Work out the finished part from the listing and answer in its coordinate system (mm). A direction names the side the tool comes from. Coordinates: 2 decimals unless noted, no trailing zeros. Loops run counter-clockwise (first coordinate to the right, second up) from the corner with the lowest first, then second, coordinate; pieces in that order, holes last. Notation, with made-up numbers: (-35.75, -19.5) -> (-30.75, -19.5) arc R33 cw to (-30.75, 16.5) -> close; hole circle Ø6 at (86, 25.25). An arc over 180 degrees is marked (long way). Use a Markdown table: item, result.
from build123d import *

# Parameters (mm, degrees)
SKETCH_R   = 11
SKETCH_R_2 = 2.5
PAD_DEPTH  = 1.3


with BuildPart() as part:
    # Sketch → Pad (new body)
    with BuildSketch(Plane.XY):
        with BuildLine():
            ThreePointArc((37.406136, 46.912482), (0, 60), (-37.406136, 46.912482))
            Line((-37.406136, 46.912482), (-31.633101, 40.032448))
            ThreePointArc((-33.931235, 38.104085), (-29.889624, 35.621067), (-31.633101, 40.032448))
            Line((-33.931235, 38.104085), (-39.704269, 44.98412))
            ThreePointArc((-39.704269, 44.98412), (0, -60), (39.704269, 44.98412))
            Line((33.931235, 38.104085), (39.704269, 44.98412))
            ThreePointArc((31.633101, 40.032448), (29.889624, 35.621067), (33.931235, 38.104085))
            Line((31.633101, 40.032448), (37.406136, 46.912482))
        make_face()
        Circle(SKETCH_R, mode=Mode.SUBTRACT)
        with Locations((0, 49)):
            Circle(SKETCH_R_2, mode=Mode.SUBTRACT)
        with Locations((48.25558, 8.508761)):
            Circle(SKETCH_R_2, mode=Mode.SUBTRACT)
        with Locations((42.435245, -24.5)):
            Circle(SKETCH_R_2, mode=Mode.SUBTRACT)
        with Locations((16.758987, -46.044938)):
            Circle(SKETCH_R_2, mode=Mode.SUBTRACT)
        with Locations((-16.758987, -46.044938)):
            Circle(SKETCH_R_2, mode=Mode.SUBTRACT)
        with Locations((-42.435245, -24.5)):
            Circle(SKETCH_R_2, mode=Mode.SUBTRACT)
        with Locations((-48.25558, 8.508761)):
            Circle(SKETCH_R_2, mode=Mode.SUBTRACT)
    extrude(amount=PAD_DEPTH)


solid = part.part
Q1. Section D-D on z = 0.35 is taken. State how many separate pieces and enclosed holes the cut face has, and give its area (3 significant figures).
Solved:
| item | result |
|---|---|
| separate pieces | 1 |
| enclosed holes | 8 |
| area | 10,700 mm² |
Q2. Section C-C on y = 43 is taken. Determine the outline of the cut face in (x, z), and give its area (3 significant figures).
Solved:
| item | result |
|---|---|
| outline | (-41.84, 0) -> (-38.04, 0) -> (-38.04, 1.3) -> (-41.84, 1.3) -> close; (-34.12, 0) -> (34.12, 0) -> (34.12, 1.3) -> (-34.12, 1.3) -> close; (38.04, 0) -> (41.84, 0) -> (41.84, 1.3) -> (38.04, 1.3) -> close |
| area | 98.6 mm² |
Q3. Determine the mould class of faces 1 (the cylindrical face through (-14.45, -47, 0.64)), 2 (the flat face through (12, 1, 0)), 3 (the cylindrical face through (0.565, 59.997, 0.641)) for opening direction Y: pulls with the +Y half, pulls with the -Y half, needs draft (parallel to the pull), parting line crosses it, or undercut.
Solved:
| item | result |
|---|---|
| face 1 | undercut |
| face 2 | needs draft |
| face 3 | pulls with the +Y half |
Q4. Section A-A on y = 0 is taken. Determine the outline of the cut face in (x, z).
Solved:
| item | result |
|---|---|
| outline | (-60, 0) -> (-11, 0) -> (-11, 1.3) -> (-60, 1.3) -> close; (11, 0) -> (60, 0) -> (60, 1.3) -> (11, 1.3) -> close |
Q5. Section B-B on x = 0 is taken. Determine the outline of the cut face in (y, z).
Solved:
| item | result |
|---|---|
| outline | (-60, 0) -> (-11, 0) -> (-11, 1.3) -> (-60, 1.3) -> close; (11, 0) -> (46.5, 0) -> (46.5, 1.3) -> (11, 1.3) -> close; (51.5, 0) -> (60, 0) -> (60, 1.3) -> (51.5, 1.3) -> close |
Q6. For faces 4 (the flat face through (-34.56, 43.52, 0.64)), 5 (the flat face through (12, 1, 1.3)), determine the directions among +Z, -Z, +X, -X, +Y, -Y from which every point of the face is accessible in a straight line to the end or side of a thin tool.
Solved:
| item | result |
|---|---|
| face 4 | +Z, -Z |
| face 5 | +Z, +X, -X, +Y, -Y |
Q7. Given pin 1 Ø4.5 at (x, y) = (-16.76, -46.04) entering from -Z, flat-ended and moving along its own axis, determine where the tip first touches the part or whether it passes through.
Solved:
| item | result |
|---|---|
| pin 1 | through |
Q8. Consider line 1 (X direction, y = -47.5, z = 0.9); line 2 (Y direction, x = 0, z = 0.75); line 3 (X direction, y = 9.5, z = 1.25). Determine where each line is inside the solid, lowest interval first. Write a range as [from, to].
Solved:
| item | result |
|---|---|
| line 1 | [-36.66, -18.79], [-14.73, 14.73], [18.79, 36.66] |
| line 2 | [-60, -11], [11, 46.5], [51.5, 60] |
| line 3 | [-59.24, -50.55], [-45.96, -5.55], [5.55, 45.96], [50.55, 59.24] |
